Here's the drawing with two shaded views (mm, measured from the low corner). I have some questions. A direction names the side the tool comes from. Coordinates: 2 decimals unless noted, no trailing zeros. Write each loop counter-clockwise with the first axis right and the second up, starting at its lowest first coordinate (ties: lowest second). Pieces come first, ordered by that corner, then holes.
Item 1: For the marked faces 5 and 6, which set-ups out of +Z, -Z, +X, -X, +Y, -Y let a thin tool reach every point of the face, with its end or its side?
Item 2: If we section it at B-B (z = 11.5): Please give me the cut outline in (x, y).
Item 3: If we section it at A-A (x = 27): Please give me the cut outline in (y, z).
Item 4: If I drill on line 1 (X direction, y = 2.9, z = 64.5); line 2 (Z direction, x = 29.5, y = 1.4); line 3 (Y direction, x = 20.5, z = 9), over which ranges is the centre line in solid material (lowest first)?
Item 5: If we section it at D-D (y = 17.5): Please give me the cut outline in (x, z), then the cut area to 3 significant figures.
Item 6: If we section it at C-C (y = 5.25): Please give me the cut outline in (x, z), then the cut area to 3 significant figures.
Item 7: We'd pull the mould along Y, two halves only. Please class the marked faces 1, 2, 3 and 4: +Y half, -Y half, draft (parallel to the pull), parting line (faces both ways), or undercut.
Item 8: I'm going to push flat-ended pins straight in: pin 1 Ø12 at (y, z) = (6, 14) entering from -X; pin 2 Ø3 at (x, z) = (35.5, 64.5) entering from +Y; pin 3 Ø6.5 at (y, z) = (14, 10.5) entering from +X; pin 4 Ø3.5 at (x, z) = (35.5, 33.5) entering from +Y. Where does each tip first touch, or does it pass through?
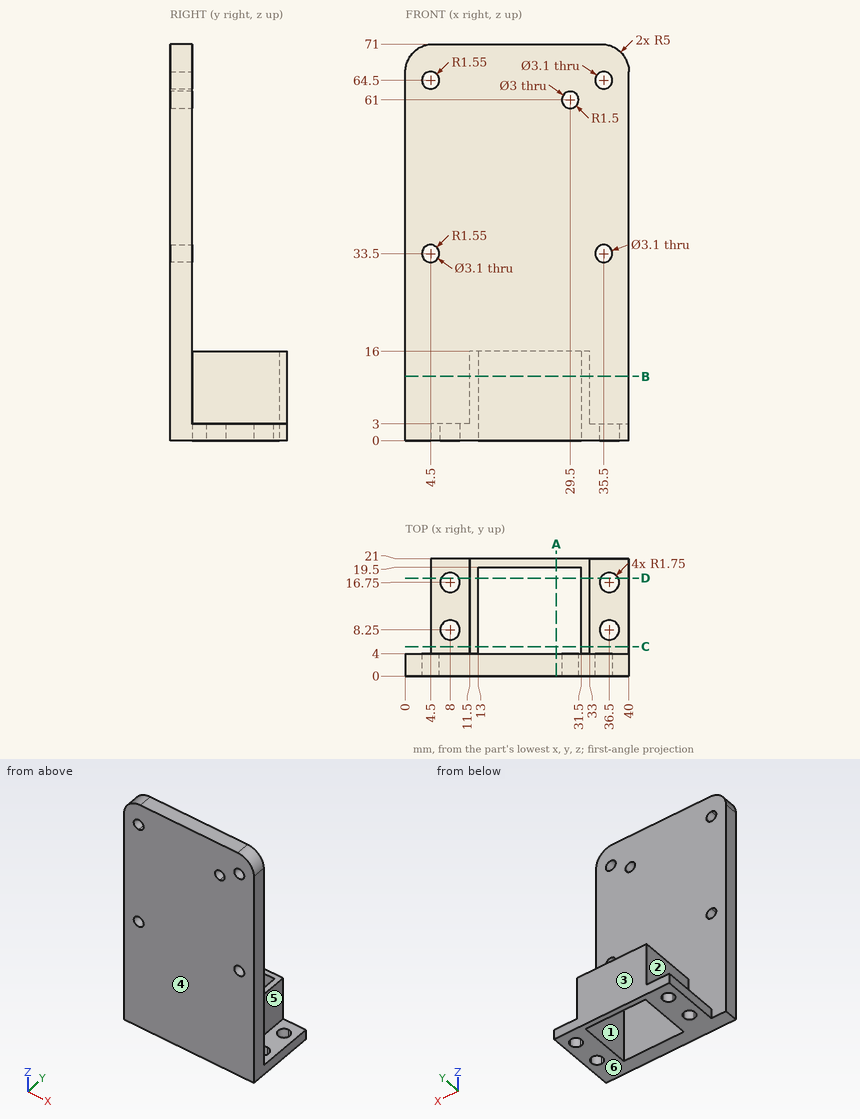
Answer list:
1. face 5: +Z, +X, +Y
1. face 6: -Z, +X, -X, +Y, -Y
2. outline: (0, 0) - (40, 0) - (40, 4) - (33, 4) - (33, 21) - (11.5, 21) - (11.5, 4) - (0, 4) - close; hole (13, 4) - (31.5, 4) - (31.5, 19.5) - (13, 19.5) - close
3. outline: (0, 0) - (4, 0) - (4, 71) - (0, 71) - close; (19.5, 0) - (21, 0) - (21, 16) - (19.5, 16) - close
4. line 1: x = 0 to 2.95, 6.05 to 33.95, 37.05 to 40
4. line 2: z = 0 to 59.5, 62.5 to 71
4. line 3: y = 0 to 4, 19.5 to 21
5. outline: (4.5, 0) - (6.42, 0) - (6.42, 3) - (4.5, 3) - close; (9.58, 0) - (13, 0) - (13, 16) - (11.5, 16) - (11.5, 3) - (9.58, 3) - close; (31.5, 0) - (34.92, 0) - (34.92, 3) - (33, 3) - (33, 16) - (31.5, 16) - close; (38.08, 0) - (40, 0) - (40, 3) - (38.08, 3) - close
5. area: 71.0 mm2
6. outline: (4.5, 0) - (13, 0) - (13, 16) - (11.5, 16) - (11.5, 3) - (4.5, 3) - close; (31.5, 0) - (40, 0) - (40, 3) - (33, 3) - (33, 16) - (31.5, 16) - close
6. area: 90.0 mm2
7. face 1: undercut
7. face 2: draft
7. face 3: +Y half
7. face 4: -Y half
8. pin 1: stops at x = 0
8. pin 2: passes through
8. pin 3: stops at x = 33
8. pin 4: stops at y = 4
